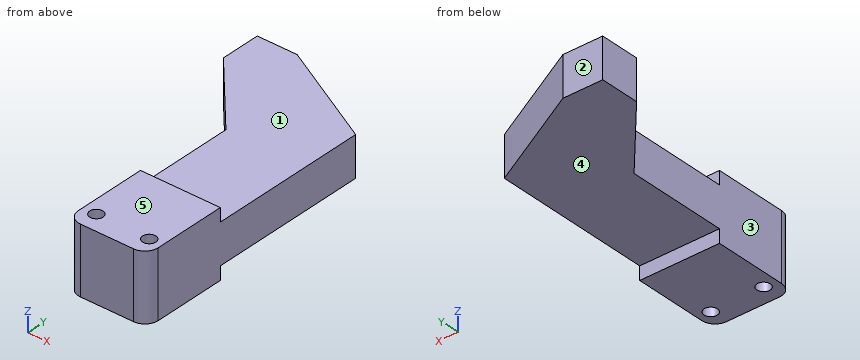
from build123d import *

# Parameters (mm, degrees)
EXTRUDE_1_DEPTH     = 9
EXTRUDE_2_DEPTH     = 36
SKETCH_3_W          = 36
SKETCH_3_H          = 39
EXTRUDE_4_DEPTH     = 15
SKETCH_5_R          = 3
CUT_EXTRUDE_1_DEPTH = 122.11819461
FILLET_1_R          = 6


with BuildPart() as part:
    # 草图1 → 凸台-拉伸1 (new, symmetric)
    with BuildSketch(Plane.XY):
        Polygon((0, 0), (0, 72), (-47.770032799, 97.179832534), (-65.770032799, 97.179832534), (-65.770032799, 79.179832534), (-36, 45.434534385), (-36, 0), align=None)
    extrude(amount=EXTRUDE_1_DEPTH, both=True)

    # 草图2 → 凸台-拉伸2 (add)
    with BuildSketch(Plane(origin=(0, 0, 0), x_dir=(0, 0, -1), z_dir=(1, 0, 0))):
        Polygon((-3.6, 0), (-8.977776638, -6), (9.022223362, -6), (3.6, 0), align=None)
    extrude(amount=-EXTRUDE_2_DEPTH)

    # 草图3 → 凸台-拉伸4 (add, symmetric)
    with BuildSketch(Plane.XY):
        with Locations((-18, -19.5)):
            Rectangle(SKETCH_3_W, SKETCH_3_H)
    extrude(amount=EXTRUDE_4_DEPTH, both=True)

    # 草图5 → 切除-拉伸1 (cut, through all)
    with BuildSketch(Plane.XY.offset(15)):
        with Locations((-29.881296057, -30.673800583)):
            Circle(SKETCH_5_R)
        with Locations((-5.88176625, -30.824030402)):
            Circle(SKETCH_5_R)
    extrude(amount=-CUT_EXTRUDE_1_DEPTH, mode=Mode.SUBTRACT)

    # 圆角1
    fillet_1_edges = [part.edges().sort_by_distance(p)[0] for p in [
        (-36, -39, 0),
        (0, -39, 0),
    ]]
    fillet(fillet_1_edges, radius=FILLET_1_R)


solid = part.part
Could you check a few things on this model? Use its own coordinates, in mm. Face numbers are marked on the shaded views. A direction names the side the tool comes from. Give positions to 0.01 mm unless a question says otherwise; leave off trailing zeros. Order: outer loops, then holes, each group sorted by start corner. A loop starts at its lowest first (then second) coordinate and runs counter-clockwise, first axis right, second up. Notation, with made-up numbers: (-39.5, 45) -> (3.5, 45) arc R25 ccw to (3.5, 60) -> close; hole circle Ø2 at (80, 28). An arc over 180 degrees is marked (long way). Return JSON: item names as keys, results as strings.
1. On a 3-axis mill with a long thin cutter (end or side, diameter ignored), from which of +Z, -Z, +X, -X, +Y, -Y can I reach the whole of each face in a straight line? I mean the marked faces 1, 2, 3, 4 and 5. Say none if no direction works.
Answer list:
{"face 1": "+Z, +X, -X, +Y", "face 2": "+Z, -Z, +X, -X, +Y", "face 3": "+Z, -Z, -X, -Y", "face 4": "-Z, +X, -X, +Y", "face 5": "+Z, +X, -X, +Y, -Y"}
2. Imagine slicing it at D-D on x = -61. List the corners of the cut face in (y, z) for me.
Answer list:
{"outline": "(73.77, -9) -> (97.18, -9) -> (97.18, 9) -> (73.77, 9) -> close"}
3. I need wall thicknesses on line 1 (Y direction, x = -5.5, z = 13.25); line 2 (Z direction, x = -5.5, y = 22); line 3 (Y direction, x = -10, z = 13.5). Which ranges of each line are inside material? Lowest first, please. Write a range as from..to.
Answer list:
{"line 1": "y = -38.98..-33.8, -27.85..0", "line 2": "z = -9..9", "line 3": "y = -39..0"}
4. Imagine slicing it at C-C on z = -11.25. List the corners of the cut face in (x, y) for me, then the cut area to 3 significant figures.
Answer list:
{"outline": "(-36, -33) arc R6 ccw to (-30, -39) -> (-6, -39) arc R6 ccw to (0, -33) -> (0, 0) -> (-36, 0) -> close; hole circle Ø6 at (-29.88, -30.67); hole circle Ø6 at (-5.88, -30.82)", "area": "1,330 mm2"}
5. Imagine slicing it at B-B on y = 35. List the corners of the cut face in (x, z) for me.
Answer list:
{"outline": "(-36, -9) -> (0, -9) -> (0, 9) -> (-36, 9) -> close"}
6. For pin 1 Ø1.5 at (y, z) = (45, 11) entering from +X; pin 2 Ø10 at (x, y) = (-33, 66) entering from +Z; pin 3 Ø4 at (x, z) = (-10, -1) entering from +Y; pin 4 Ø1.8 at (x, z) = (-21, 11) entering from +Y, each with a flat end and sliding along its axis, tell me the tip position at first contact or that it passes through.
Answer list:
{"pin 1": "passes through", "pin 2": "stops at z = 9", "pin 3": "stops at y = 78.33", "pin 4": "stops at y = 0"}
7. Imagine slicing it at A-A on z = 6.5. List the corners of the cut face in (x, y) for me, then the cut area to 3 significant figures.
Answer list:
{"outline": "(-65.77, 79.18) -> (-36, 45.43) -> (-36, -33) arc R6 ccw to (-30, -39) -> (-6, -39) arc R6 ccw to (0, -33) -> (0, 72) -> (-47.77, 97.18) -> (-65.77, 97.18) -> close; hole circle Ø6 at (-29.88, -30.67); hole circle Ø6 at (-5.88, -30.82)", "area": "5,270 mm2"}
